Check sheet for the modelled part. Datum: model origin and axes. Units: mm. Face numbers are marked on the shaded views. Round coordinates to 2 decimals unless told otherwise and drop trailing zeros. Write each loop counter-clockwise with the first axis right and the second up, starting at its lowest first coordinate (ties: lowest second). Pieces come first, ordered by that corner, then holes. Notation, with made-up numbers: (11.25, 75) - (29.25, 75) arc R19 cw to (29.25, 85) - close; hole circle Ø8 at (-0.5, 75). An arc over 180 degrees is marked (long way). Use one line per item in the form item = value. Start each with the question number.
1) Draft check along X on the marked faces 1, 2 and 3. Enter one of: +X half, -X half, draft (parallel to the pull), parting line (faces both ways), or undercut.
2) Scan lines: probe 1 along Z at (x, y) = (0, 2.95); probe 2 along Y at (x, z) = (-1.25, 3); probe 3 along X at (y, z) = (-3, 0). Record each from-to range of solid material in increasing order.
3) Section check C-C (z = 0). Record the boundary of the cut face in (x, y).
4) Section check B-B (y = 0). Record the boundary of the cut face in (x, z), then the cut area to 3 significant figures.
5) Section check A-A (x = 0). Record the boundary of the cut face in (y, z).
6) Gauge pin test, flat ends, axial feed: P1, Ø3, axis at y = 2.5, z = 0.5, coming from the -X side; P2, Ø1.5, axis at y = -2, z = 1, coming from the -X side. Record the tip position at first contact, or that the pin passes through.
7) Section check D-D (z = -3.5). Record the boundary of the cut face in (x, y).
Autodesk Inventor part; units mm, degrees
ref_plane "Work Plane1" through (0, 4, 0) normal (0, 1, 0) x (-1, 0, 0)
ref_plane "YZ Plane" through (0, 0, 0) normal (1, 0, 0) x (0, 1, 0)
ref_plane "XY Plane" through (0, 0, 0) normal (0, 0, 1) x (1, 0, 0)
sketch "Sketch1" plane through (0, 0, 0) normal (0, 0, 1) x (1, 0, 0)
  circle A0 centre (0, 0) radius 4
  circle A1 centre (0, 0) radius 2.5
  dimension "d0" = 8
  dimension "d1" = 5
extrude "Extrusion1" add sketch "Sketch1" along normal mid plane 8
ref_plane "Work Plane1" through (0, 4, 0) normal (0, 1, 0) x (-1, 0, 0)
sketch "Sketch2" plane through (0, 4, 0) normal (0, 1, 0) x (-1, 0, 0)
  point P0 (0, 0)
  point P1 (0, 0)
hole "Hole1" at (0, 4, 0) direction (0, -1, 0) diameter 2.5 depth 8
properties part number "10.1"
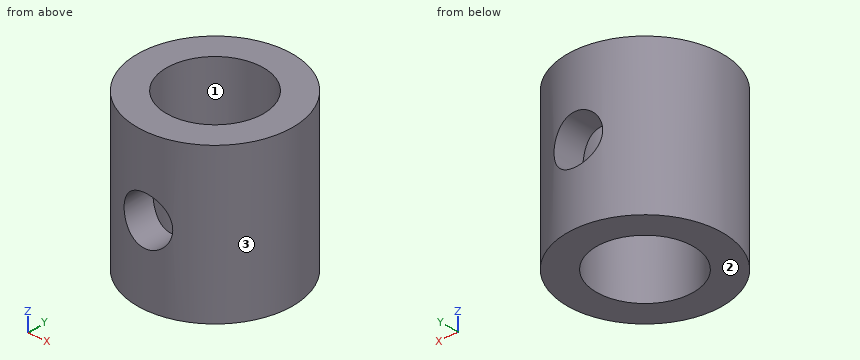
Results are:
q1.face_1 = undercut
q1.face_2 = draft
q1.face_3 = parting line
q2.probe_1 = -4 to -1.25, 1.25 to 4
q2.probe_2 = -3.8 to -2.17, 2.17 to 3.8
q2.probe_3 = -2.65 to -1.25, 1.25 to 2.65
q3.outline = (-1.25, -3.8) - (-1.25, -2.17) arc R2.5 cw to (-1.25, 2.17) - (-1.25, 3.8) arc R4 ccw to start; (1.25, -3.8) arc R4 ccw to (1.25, 3.8) - (1.25, 2.17) arc R2.5 cw to (1.25, -2.17) - close
q4.outline = (-4, -4) - (-2.5, -4) - (-2.5, 4) - (-4, 4) - close; (2.5, -4) - (4, -4) - (4, 4) - (2.5, 4) - close
q4.area = 24.0 mm²
q5.outline = (-4, -4) - (-2.5, -4) - (-2.5, -1.25) - (-4, -1.25) - close; (-4, 1.25) - (-2.5, 1.25) - (-2.5, 4) - (-4, 4) - close; (2.5, -4) - (4, -4) - (4, -1.25) - (2.5, -1.25) - close; (2.5, 1.25) - (4, 1.25) - (4, 4) - (2.5, 4) - close
q6.P1 = -3.87
q6.P2 = -3.8
q7.outline = circle Ø8 at (0, 0); hole circle Ø5 at (0, 0)
